Read the model definition and answer for the solid it produces. Units are mm, in the model's axes. A direction names the side the tool comes from. Coordinates: 2 decimals unless noted, no trailing zeros. Write each loop counter-clockwise with the first axis right and the second up, starting at its lowest first coordinate (ties: lowest second). Pieces come first, ordered by that corner, then holes. Notation, with made-up numbers: (41.5, 11.25) -> (69.5, 11.25) arc R24 cw to (69.5, 26.25) -> close; hole circle Ø4 at (22.25, 38.5). An arc over 180 degrees is marked (long way). Use CSV: the item, a comma, the result in double quotes.
Autodesk Inventor part; units mm, degrees
ref_plane "YZ Plane" through (0, 0, 0) normal (1, 0, 0) x (0, 1, 0)
ref_plane "XZ Plane" through (0, 0, 0) normal (0, 1, 0) x (-1, 0, 0)
ref_plane "XY Plane" through (0, 0, 0) normal (0, 0, 1) x (1, 0, 0)
sketch "Sketch1" plane through (0, 0, 0) normal (0, 0, 1) x (1, 0, 0)
  arc A0 (-4.445, 0) -> (4.445, 0) centre (0, 0) ccw
  line L0 (-4.445, 0) -> (-4.445, 8.89)
  line L1 (-4.445, 8.89) -> (4.445, 8.89)
  line L2 (4.445, 8.89) -> (4.445, 0)
  arc A1 (4.445, 0) -> (-4.445, 0) centre (0, 0) ccw construction
  dimension "d0" = 8.89
  dimension "d1" = 8.89
sketch "Sketch1 outline for Extrusion1" plane through (0, 0, 0) normal (0, 0, 1) x (1, 0, 0)
  line L0 (-4.445, 8.89) -> (-4.445, 0)
  line L1 (4.445, 8.89) -> (-4.445, 8.89)
  line L2 (4.445, 0) -> (4.445, 8.89)
  arc A0 (-4.445, 0) -> (4.445, 0) centre (0, 0) ccw
extrude "Extrusion1" add sketch "Sketch1 outline for Extrusion1" along normal mid plane 5.715
sketch "Sketch2" plane through (0, 0, 2.8575) normal (0, 0, 1) x (1, 0, 0)
  arc A0 (1.651, -1.184577) -> (-1.651, -1.184577) centre (0, 0) ccw
  line L0 (1.651, -1.184577) -> (1.905, -4.016093)
  line L1 (0, 0) -> (0, -4.445) construction
  line L2 (-1.651, -1.184577) -> (-1.905, -4.016093)
  arc A1 (0, -2.032) -> (1.651, -1.184577) centre (0, 0) ccw construction
  arc A2 (-1.651, -1.184577) -> (0, -2.032) centre (0, 0) ccw construction
  arc A3 (-4.445, 0) -> (4.445, 0) centre (0, 0) ccw
  dimension "d4" = 4.064
  dimension "d5" = 3.81
  dimension "d6" = 3.302
sketch "Sketch2 outline for Extrusion2" plane through (0, 0, 2.8575) normal (0, 0, 1) x (1, 0, 0)
  line L0 (1.905, -4.016093) -> (1.651, -1.184577)
  arc A0 (-1.905, -4.016093) -> (1.905, -4.016093) centre (0, 0) ccw
  line L1 (-1.651, -1.184577) -> (-1.905, -4.016093)
  arc A1 (1.651, -1.184577) -> (-1.651, -1.184577) centre (0, 0) ccw
extrude "Extrusion2" cut sketch "Sketch2 outline for Extrusion2" against normal through all
sketch "Sketch3" plane through (0, 0, 0) normal (0, 0, 1) x (1, 0, 0)
  line L0 (4.445, 8.89) -> (-4.445, 8.89)
  line L1 (0, 7.62) -> (4.445, 8.89)
  line L2 (4.445, 8.89) -> (8.89, 10.16)
  line L3 (8.89, 10.16) -> (8.89, 11.43)
  line L4 (8.89, 11.43) -> (7.62, 11.43)
  line L5 (7.62, 11.43) -> (7.62, 15.24)
  line L6 (7.62, 15.24) -> (0, 15.24)
  line L7 (0, 15.24) -> (0, 7.62)
  line L8 (0, 0) -> (0, 8.89) construction
  line L9 (0, -7.867311) -> (0, 19.091219)
  dimension "d9" = 8.89
  dimension "d10" = 6.35
  dimension "d11" = 3.81
  dimension "d12" = 1.27
  dimension "d13" = 1.27
sketch "Sketch3 outline for Revolution1" plane through (0, 0, 0) normal (0, 0, 1) x (1, 0, 0)
  line L0 (0, 15.24) -> (0, 7.62)
  line L1 (7.62, 15.24) -> (0, 15.24)
  line L2 (7.62, 11.43) -> (7.62, 15.24)
  line L3 (8.89, 11.43) -> (7.62, 11.43)
  line L4 (8.89, 10.16) -> (8.89, 11.43)
  line L5 (4.445, 8.89) -> (8.89, 10.16)
  line L6 (0, 7.62) -> (4.445, 8.89)
revolve "Revolution1" add sketch "Sketch3 outline for Revolution1" angle 360 about axis through (0, -10, 0) along (0, 1, 0)
sketch "Sketch4" plane through (0, 15.24, 0) normal (0, 1, 0) x (1, 0, 0)
  circle A0 centre (0, 0) radius 3.175
  circle A1 centre (0, 0) radius 7.62
  circle A2 centre (0, 0) radius 6.35
  dimension "d15" = 6.35
  dimension "d16" = 1.27
sketch "Sketch4 outline for Extrusion3" plane through (0, 15.24, 0) normal (0, 1, 0) x (1, 0, 0)
  circle A0 centre (0, 0) radius 6.35
  circle A1 centre (0, 0) radius 3.175
extrude "Extrusion3" cut sketch "Sketch4 outline for Extrusion3" against normal blind 2.54
sketch "Sketch5" plane through (0, 15.24, 0) normal (0, 1, 0) x (1, 0, 0)
  circle A0 centre (0, 0) radius 1.5875
  dimension "d19" = 3.175
sketch "Sketch5 outline for Extrusion4" plane through (0, 15.24, 0) normal (0, 1, 0) x (1, 0, 0)
  circle A0 centre (0, 0) radius 1.5875
extrude "Extrusion4" add sketch "Sketch5 outline for Extrusion4" along normal blind 35.56
properties part number "Bottom"
1. A tool of negligible diameter and unlimited length cuts with its end or side. For faces 4 (the flat face through (4.445, 4, 0)), 5 (the flat face through (-4.445, 5, 0)), 6 (the cylindrical face through (-0.69, 13.99, 3.1)), from which of +Z, -Z, +X, -X, +Y, -Y can it reach the whole face along a straight path? Write none if from no direction.
Solutions:
face 4,"+Z, -Z, +X, -Y"
face 5,"+Z, -Z, -X, -Y"
face 6,"+Y"
2. For a pull along Y with two mould halves and no side action, classify faces 1 (the cylindrical face through (0.06, 2.03, 0.04)), 2 (the cylindrical face through (-1.38, 13.99, 6.2)), 3 (the flat face through (1.78, -2.62, 0.04)) as pulls with the +Y half, pulls with the -Y half, needs draft (parallel to the pull), parting line crosses it, or undercut.
Solutions:
face 1,"undercut"
face 2,"needs draft"
face 3,"pulls with the -Y half"
3. A cutting plane is placed at A-A (y = 38). Give the vertices of the cut face in (x, z) (1 decimal), and give its area (3 significant figures).
Solutions:
outline,"circle Ø3.2 at (0, 0)"
area,"7.92 mm^2"
4. Each of these flat-tipped pins is pushed along its axis until it touches: pin 1 Ø10 at (x, y) = (2, 1) entering from -Z; pin 2 Ø0.8 at (x, z) = (4, -1.5) entering from +Y; pin 3 Ø1.5 at (x, z) = (7, 5.5) entering from -Y. Where does it stop, or does it pass through?
Solutions:
pin 1,"stops at z = -2.86"
pin 2,"stops at y = 12.7"
pin 3,"stops at y = 9.95"
5. Find the intervals of material crossed by line 1 along X through (y, z) = (13.8, 0) (3 decimals); line 2 along X through (y, z) = (0, 1.65) (3 decimals); line 3 along Y through (x, z) = (0, -1.55), in increasing order.
Solutions:
line 1,"x = -7.62 to -6.35, -3.175 to 3.175, 6.35 to 7.62"
line 2,"x = -4.445 to -2.032, 2.032 to 4.445"
line 3,"y = 2.03 to 50.8"
